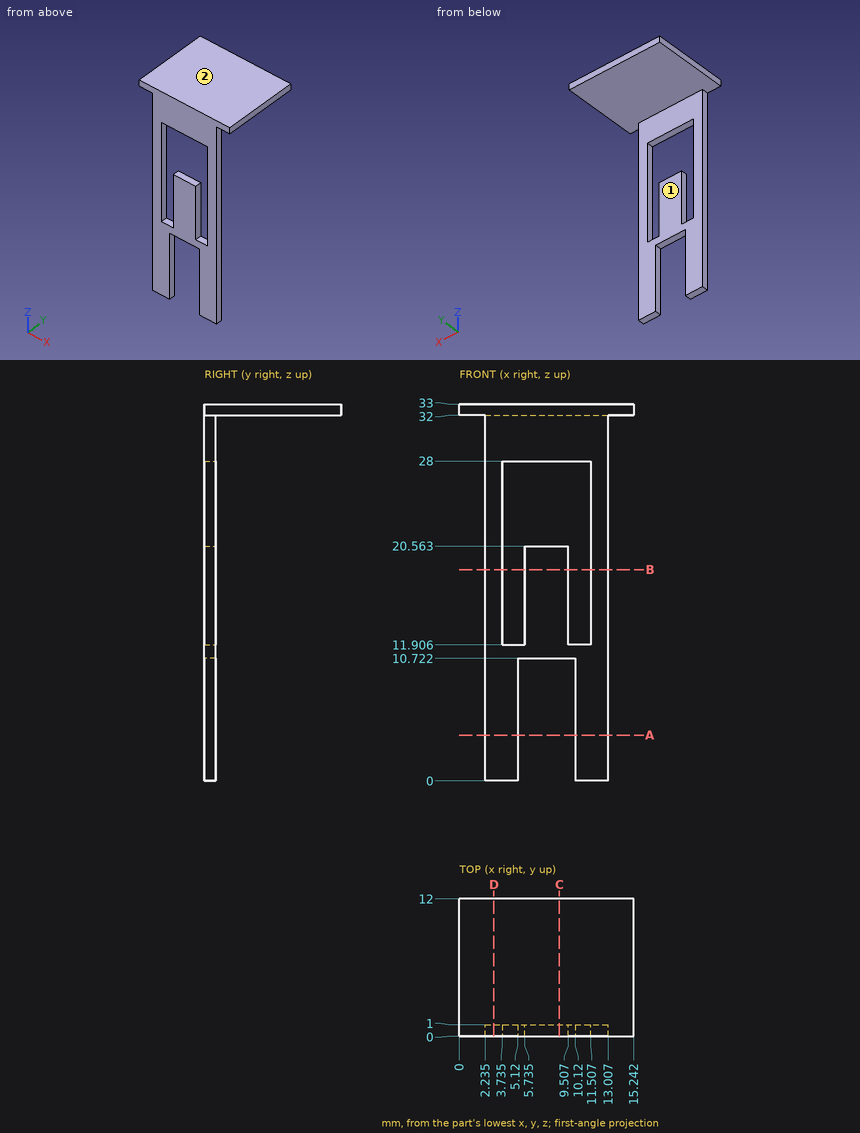
Verification items for this drawing (mm, ordinates from the low corner). A direction names the side the tool comes from. Give positions to 0.01 mm unless a question says otherwise; leave off trailing zeros. Write each loop counter-clockwise with the first axis right and the second up, starting at its lowest first coordinate (ties: lowest second). Pieces come first, ordered by that corner, then holes.
1) Thickness scan on line 1 (Z direction, x = 4, y = 0.5) (1 decimal); line 2 (Z direction, x = 12.25, y = 11); line 3 (Y direction, x = 11.75, z = 23). Record the ranges inside material, lowest first.
Values follow:
line 1: z = 0 to 11.9, 28 to 33
line 2: z = 32 to 33
line 3: y = 0 to 1
2) Set-up check for the marked faces 1 and 2: record each of +Z, -Z, +X, -X, +Y, -Y from which the full face is reachable in a straight line by a thin tool's end or side.
Values follow:
face 1: -Z, +X, -X, +Y
face 2: +Z, +X, -X, +Y, -Y
3) Cross-section at D-D (x = 3). Record the boundary of the cut face in (y, z).
Values follow:
outline: (0, 0) - (1, 0) - (1, 32) - (12, 32) - (12, 33) - (0, 33) - close
4) Cross-section at A-A (z = 4). Record the boundary of the cut face in (x, y) (1 decimal).
Values follow:
outline: (2.2, 0) - (5.1, 0) - (5.1, 1) - (2.2, 1) - close; (10.1, 0) - (13, 0) - (13, 1) - (10.1, 1) - close
5) Cross-section at C-C (x = 8.75). Record the boundary of the cut face in (y, z).
Values follow:
outline: (0, 10.72) - (1, 10.72) - (1, 20.56) - (0, 20.56) - close; (0, 28) - (1, 28) - (1, 32) - (12, 32) - (12, 33) - (0, 33) - close
6) Cross-section at B-B (z = 18.5). Record the boundary of the cut face in (x, y) (1 decimal).
Values follow:
outline: (2.2, 0) - (3.7, 0) - (3.7, 1) - (2.2, 1) - close; (5.7, 0) - (9.5, 0) - (9.5, 1) - (5.7, 1) - close; (11.5, 0) - (13, 0) - (13, 1) - (11.5, 1) - close
7) Go/stop test with flat-tipped pins: pin 1 Ø0.8 at (x, y) = (8.5, 0.5) entering from -Z; pin 2 Ø0.8 at (y, z) = (0.5, 16.5) entering from +X; pin 3 Ø3 at (x, z) = (10, 12.5) entering from +Y. Record where each tip stops, or that it passes through.
Values follow:
pin 1: stops at z = 10.72
pin 2: stops at x = 13.01
pin 3: stops at y = 1
